For this review, take the finished solid that the model builds, in its own axes (mm). Coordinates: 2 decimals unless noted, no trailing zeros. Write each loop counter-clockwise with the first axis right and the second up, starting at its lowest first coordinate (ties: lowest second). Pieces come first, ordered by that corner, then holes.
1) To check wall thickness, follow line 1 along X through (y, z) = (193.5, 18.5); line 2 along Z through (x, y) = (345.5, 187); line 3 along Z through (x, y) = (27, 214). State the ranges of each line that lie inside material, in increasing order.
2) We need section B-B on z = 15. Write out the cut boundary in (x, y), then the cut area to 3 significant figures.
3) We need section C-C on x = 36. Write out the cut boundary in (y, z), then the cut area to 3 significant figures.
4) We need section A-A on y = 118. Write out the cut boundary in (x, z).
5) Insertion check: P1, Ø1, axis at y = 190, z = 14.5, coming from the +X side; P2, Ø8, axis at y = 62.5, z = 8.5, coming from the +X side; P3, Ø12, axis at y = 134.5, z = 17.5, coming from the +X side. Each pin has a flat end and moves straight along its axis. Give the tip position at first contact, or say it passes through.
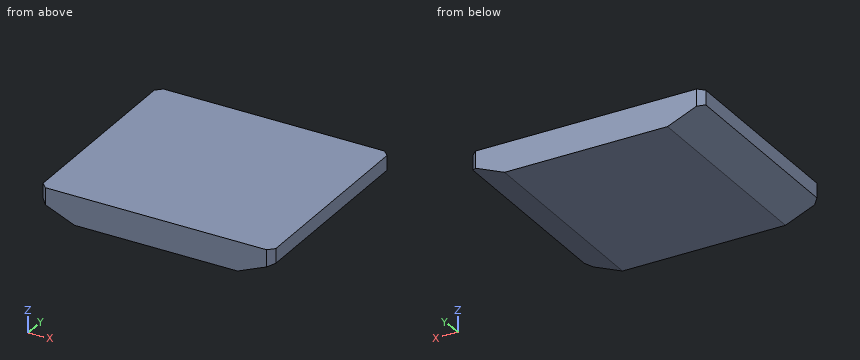
from build123d import *

# Parameters (mm, degrees)
SKETCH_W     = 400
SKETCH_H     = 350
PAD_DEPTH    = 50
POCKET_DEPTH = 350.001
CHAMFER_SIZE = 10


with BuildPart() as part:
    # Sketch → Pad (new body)
    with BuildSketch(Plane.XY):
        with Locations((200, 175)):
            Rectangle(SKETCH_W, SKETCH_H)
    extrude(amount=PAD_DEPTH)

    # Sketch001 (on Face1 of Pad) → Pocket (cut, through all)
    with BuildSketch(Plane.XZ):
        Polygon((0, 25), (60, 0), (0, 0), align=None)
        Polygon((400, 25), (340, 0), (400, 0), align=None)
    extrude(amount=-POCKET_DEPTH, mode=Mode.SUBTRACT)

    # Chamfer
    chamfer_edges = [part.edges().sort_by_distance(p)[0] for p in [
        (400, 0, 37.5),
        (0, 0, 37.5),
        (400, 350, 37.5),
        (0, 350, 37.5),
    ]]
    chamfer(chamfer_edges, length=CHAMFER_SIZE)


solid = part.part
Result:
1. line 1: x = 15.6 to 384.4
1. line 2: z = 2.29 to 50
1. line 3: z = 13.75 to 50
2. outline: (24, 0) - (376, 0) - (376, 350) - (24, 350) - close
2. area: 123,000 mm2
3. outline: (0, 10) - (350, 10) - (350, 50) - (0, 50) - close
3. area: 14,000 mm2
4. outline: (0, 25) - (60, 0) - (340, 0) - (400, 25) - (400, 50) - (0, 50) - close
5. P1: stops at x = 376
5. P2: stops at x = 370
5. P3: stops at x = 396.4
